For this review, take the finished solid that the model builds, in its own axes (mm). A direction names the side the tool comes from. Give positions to 0.01 mm unless a question says otherwise; leave off trailing zeros. Order: outer loops, then holes, each group sorted by start corner. A loop starts at its lowest first (then second) coordinate and runs counter-clockwise, first axis right, second up. Notation, with made-up numbers: (-20, 78.25) - (-7, 78.25) arc R13 cw to (-7, 95.25) - close; hole circle Ø2 at (80.25, 26). An arc over 180 degrees is marked (long way). Use a Markdown table: item, result. Add a question column.
1) We need section B-B on z = 11. Write out the cut boundary in (x, y), then the cut area to 3 significant figures.
2) We need section D-D on z = 16.75. Write out the cut boundary in (x, y), then the cut area to 3 significant figures.
3) We need section C-C on z = 3. Write out the cut boundary in (x, y), then the cut area to 3 significant figures.
4) We need section A-A on y = 0.75. Give the number of separate pieces and of enclosed holes in the cut face, then the cut area to 3 significant figures.
5) Clearance check with flat-ended pins moving along their axes: P1, Ø1.5, axis at y = 4, z = 12.5, coming from the +X side; P2, Ø3, axis at y = 3.5, z = 2.5, coming from the -X side; P3, Ø3, axis at y = 2.5, z = 5.5, coming from the -X side. State where each tip first meets the part, or that it passes through.
6) Wall thickness on L1, parallel to Z at x = -9.25, y = 3.75; L2, parallel to X at y = 0.65, z = 8.75; L3, parallel to X at y = 1.35, z = 11.75: over which ranges is each line inside the solid? List them lowest first.
7) Machinability: for faces 1 (the face through (-109.5, 2.5, 9.2)), 2 (the face through (-58, 2, 18.5)), which of the approach directions +Z, -Z, +X, -X, +Y, -Y give a long, thin tool a straight path to every point of the face, cutting with its end or side? Answer none if there is none.
8) Mouldability with a two-part tool opening along X and no side actions: class faces 3 (the face through (-56, 5, 9)), 4 (the face through (-2.78, 2.54, 15.86)), 5 (the face through (-102.5, 2.5, 9.2)) as released by +X, released by -X, zero draft, split by the parting line, or undercut.
Autodesk Inventor part; units mm, degrees
ref_plane "YZ Plane" through (0, 0, 0) normal (1, 0, 0) x (0, 1, 0)
ref_plane "XZ Plane" through (0, 0, 0) normal (0, 1, 0) x (-1, 0, 0)
ref_plane "XY Plane" through (0, 0, 0) normal (0, 0, 1) x (1, 0, 0)
sketch "Sketch1" plane through (0, 0, 0) normal (0, 1, 0) x (-1, 0, 0)
  line L0 (0, 0) -> (114.5, 0)
  line L1 (114.5, 0) -> (114.5, 18.5)
  line L2 (114.5, 18.5) -> (0, 18.5)
  line L3 (0, 18.5) -> (0, 0)
  circle A0 centre (105.25, 9.25) radius 2.75
  circle A1 centre (9.25, 9.25) radius 4.25
  dimension "d12" = 5.5
  dimension "d44" = 8.5
  dimension "d52" = 96
  dimension "d57" = 9.25
  dimension "d58" = 9.25
  dimension "d59" = 9.25
  dimension "d60" = 9.25
extrude "Extrusion3" add sketch "Sketch1" along normal blind 5
fillet "Fillet3" radius 9.25 1 edges at (-114.5, 2.5, 0)
fillet "Fillet4" radius 9.25 3 edges at (-114.5, 2.5, 18.5) (0, 2.5, 18.5) (0, 2.5, 0)
sketch "Sketch2" plane through (0, 0, 0) normal (0, -1, 0) x (1, 0, 0)
  point P0 (0, 0)
sketch "Sketch3" plane through (0, 5, 0) normal (0, 1, 0) x (1, 0, 0)
  circle A0 centre (-105.25, -9.25) radius 2.75
  circle A1 centre (-106.75, -9.25) radius 2.75
  line L0 (-106.75, -6.5) -> (-105.25, -6.5)
  line L1 (-105.25, -12) -> (-106.75, -12)
  line L2 (-106.75, -6.5) -> (-105.25, -6.5)
  line L3 (-106.75, -12) -> (-105.25, -12)
  point P0 (0, 0)
  dimension "d62" = 5.5
  dimension "d64" = 1.5
extrude "Extrusion4" cut sketch "Sketch3" against normal blind 10 contours A0 A1 L0 | L1 A1 A0 | A0 A1 picked at (-108.9803, -9.1424)
properties part number "crankRod1"
Checked values:
| question | item | result |
|---|---|---|
| 1 | outline | (-114.33, 0) - (-108.87, 0) - (-108.87, 5) - (-114.33, 5) - close; (-103.13, 0) - (-13.12, 0) - (-13.12, 5) - (-103.13, 5) - close; (-5.38, 0) - (-0.17, 0) - (-0.17, 5) - (-5.38, 5) - close |
| 1 | area | 503 mm² |
| 2 | outline | (-110.66, 0) - (-3.84, 0) - (-3.84, 5) - (-110.66, 5) - close |
| 2 | area | 534 mm² |
| 3 | outline | (-112.07, 0) - (-2.43, 0) - (-2.43, 5) - (-112.07, 5) - close |
| 3 | area | 548 mm² |
| 4 | separate pieces | 1 |
| 4 | enclosed holes | 2 |
| 4 | area | 1,960 mm² |
| 5 | P1 | x = -0.34 |
| 5 | P2 | x = -112.87 |
| 5 | P3 | x = -114.22 |
| 6 | L1 | 0 to 5, 13.5 to 18.5 |
| 6 | L2 | -114.49 to -109.45, -102.55 to -13.47, -5.03 to -0.01 |
| 6 | L3 | -114.16 to -107.9, -104.1 to -12.69, -5.81 to -0.34 |
| 7 | face 1 | +Y, -Y |
| 7 | face 2 | +Z, +X, -X, +Y, -Y |
| 8 | face 3 | zero draft |
| 8 | face 4 | released by +X |
| 8 | face 5 | undercut |
